Part model, mm, in its own coordinate system. Face numbers are marked on the shaded views. Give positions to 0.01 mm unless a question says otherwise; leave off trailing zeros. Order: outer loops, then holes, each group sorted by start corner. A loop starts at its lowest first (then second) coordinate and runs counter-clockwise, first axis right, second up. Notation, with made-up numbers: M -17,52 L 32,52 A29 ccw 32,75 Z; hole C 62,-31 d10. An arc over 180 degrees is marked long. Answer as a JSON object with one key per item and string values.
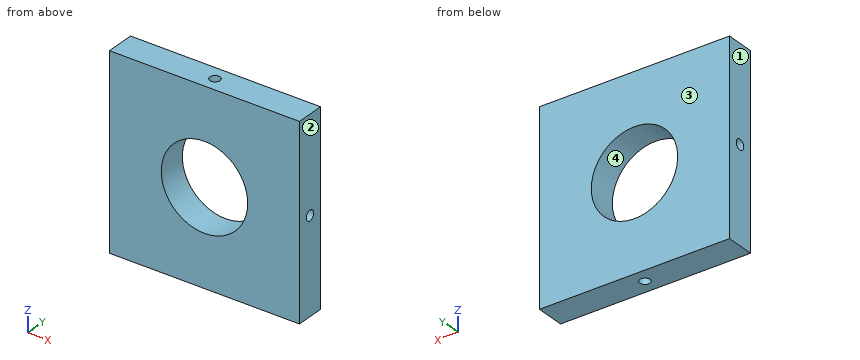
from build123d import *

# Parameters (mm, degrees)
SKETCH1_W                 = 33
SKETCH1_H                 = 33
SKETCH1_R                 = 7.5
BOSS_EXTRUDE1_DEPTH       = 5
F_2_56_TAPPED_HOLE4_D     = 1.778
F_2_56_TAPPED_HOLE4_DEPTH = 6.46583491
F_2_56_TAPPED_HOLE4_TIP   = 0.53416509
F_2_56_TAPPED_HOLE5_D     = 1.778
F_2_56_TAPPED_HOLE5_DEPTH = 7.46583491
F_2_56_TAPPED_HOLE5_TIP   = 0.53416509
F_2_56_TAPPED_HOLE6_D     = 1.778
F_2_56_TAPPED_HOLE6_DEPTH = 7.46583491
F_2_56_TAPPED_HOLE6_TIP   = 0.53416509
F_2_56_TAPPED_HOLE7_D     = 1.778
F_2_56_TAPPED_HOLE7_DEPTH = 7.46583491
F_2_56_TAPPED_HOLE7_TIP   = 0.53416509


with BuildPart() as part:
    # Sketch1 → Boss-Extrude1 (new body)
    with BuildSketch(Plane(origin=(0, 0, 0), x_dir=(1, 0, 0), z_dir=(0, 1, 0))):
        Rectangle(SKETCH1_W, SKETCH1_H)
        Circle(SKETCH1_R, mode=Mode.SUBTRACT)
    extrude(amount=BOSS_EXTRUDE1_DEPTH)

    # #2-56 Tapped Hole4
    with Locations(Plane.XY.offset(16.5)):
        with Locations((0, 2.5)):
            Hole(F_2_56_TAPPED_HOLE4_D / 2, depth=F_2_56_TAPPED_HOLE4_DEPTH)
            with Locations((0, 0, -(F_2_56_TAPPED_HOLE4_DEPTH + F_2_56_TAPPED_HOLE4_TIP / 2))):  # 118° drill point
                Cone(0, F_2_56_TAPPED_HOLE4_D / 2, F_2_56_TAPPED_HOLE4_TIP, mode=Mode.SUBTRACT)

    # #2-56 Tapped Hole5
    with Locations(Plane(origin=(0, 0, -16.5), x_dir=(-1, 0, 0), z_dir=(0, 0, -1))):
        with Locations((0, 2.5)):
            Hole(F_2_56_TAPPED_HOLE5_D / 2, depth=F_2_56_TAPPED_HOLE5_DEPTH)
            with Locations((0, 0, -(F_2_56_TAPPED_HOLE5_DEPTH + F_2_56_TAPPED_HOLE5_TIP / 2))):  # 118° drill point
                Cone(0, F_2_56_TAPPED_HOLE5_D / 2, F_2_56_TAPPED_HOLE5_TIP, mode=Mode.SUBTRACT)

    # #2-56 Tapped Hole6
    with Locations(Plane(origin=(16.5, 0, 0), x_dir=(0, 0, -1), z_dir=(1, 0, 0))):
        with Locations((0, 2.5)):
            Hole(F_2_56_TAPPED_HOLE6_D / 2, depth=F_2_56_TAPPED_HOLE6_DEPTH)
            with Locations((0, 0, -(F_2_56_TAPPED_HOLE6_DEPTH + F_2_56_TAPPED_HOLE6_TIP / 2))):  # 118° drill point
                Cone(0, F_2_56_TAPPED_HOLE6_D / 2, F_2_56_TAPPED_HOLE6_TIP, mode=Mode.SUBTRACT)

    # #2-56 Tapped Hole7
    with Locations(Plane.ZY.offset(16.5)):
        with Locations((0, 2.5)):
            Hole(F_2_56_TAPPED_HOLE7_D / 2, depth=F_2_56_TAPPED_HOLE7_DEPTH)
            with Locations((0, 0, -(F_2_56_TAPPED_HOLE7_DEPTH + F_2_56_TAPPED_HOLE7_TIP / 2))):  # 118° drill point
                Cone(0, F_2_56_TAPPED_HOLE7_D / 2, F_2_56_TAPPED_HOLE7_TIP, mode=Mode.SUBTRACT)


solid = part.part
1. Two-plate mould, pull along X, no slides. Class the marked faces 1, 2, 3 and 4: +X half, -X half, draft (parallel to the pull), parting line (faces both ways), or undercut.
Worked answers:
{"face 1": "-X half", "face 2": "+X half", "face 3": "draft", "face 4": "undercut"}
2. Cut at B-B on y = 4.6. Give the cut face in (x, z), plus the area to 3 significant figures.
Worked answers:
{"outline": "M -16.5,-16.5 L 16.5,-16.5 L 16.5,16.5 L -16.5,16.5 Z; hole C 0,0 d15", "area": "912 mm^2"}
3. Cut at A-A on x = 7. Give the cut face in (y, z).
Worked answers:
{"outline": "M 0,-16.5 L 5,-16.5 L 5,-2.69 L 0,-2.69 Z; M 0,2.69 L 5,2.69 L 5,16.5 L 0,16.5 Z"}
4. Cut at C-C on x = -12.5. Give the cut face in (y, z), plus the area to 3 significant figures.
Worked answers:
{"outline": "M 0,-16.5 L 5,-16.5 L 5,16.5 L 0,16.5 Z; hole C 2.5,0 d1.78", "area": "163 mm^2"}
5. Probe line 1 along Z through (x, y) = (14.5, 2.5); line 2 along Y through (x, z) = (13.75, 0). List the from-to ranges inside material, lowest first.
Worked answers:
{"line 1": "z = -16.5 to -0.89, 0.89 to 16.5", "line 2": "y = 0 to 1.61, 3.39 to 5"}
6. Cut at D-D on z = 3. Give the cut face in (x, y).
Worked answers:
{"outline": "M -16.5,0 L -6.87,0 L -6.87,5 L -16.5,5 Z; M 6.87,0 L 16.5,0 L 16.5,5 L 6.87,5 Z"}
7. Pin check, flat tips, straight feed: P1, Ø2.5, axis at x = 0, y = 2.5, coming from the -Z side; P2, Ø1.4, axis at x = 0, y = 2.5, coming from the -Z side; P3, Ø1.6, axis at y = 2.5, z = 0, coming from the -X side. Stop position of each tip, or through.
Worked answers:
{"P1": "stops at z = -16.5", "P2": "stops at z = -8.92", "P3": "stops at x = -8.98"}
